from build123d import *

# Parameters (mm, degrees)
F1_DEPTH    = 16
F2_T        = 3
F2_T3_DEPTH = 22
F3_R        = 7.99999
F4_R        = 3.1035458613
F4_R_2      = 3.5498541614
F5_DEPTH    = 20


# Not quite as in the source:
# - a fillet or chamfer is up to 0.001 mm smaller than in the source, because OpenCascade refuses the exact size
# - a shell that OpenCascade refuses in one call is made with other operations: the cavity is built on its own and cut out


with BuildPart() as f1:
    # F0 (on Front) → F1 (new body)
    with BuildSketch(Plane.XZ):
        Polygon((-64.2090581298, 10), (-64.2090581298, 0), (31.7909418702, 0), (29.6909418702, 3), (24.7909418702, 10), (0.7909418702, 10), (-7.2090581298, 14), (-42.2090581298, 14), (-50.2090581298, 10), align=None)
        Polygon((31.7909418702, 0), (-64.2090581298, 0), (-64.2090581298, -10), (-50.2090581298, -10), (-42.2090581298, -14), (-7.2090581298, -14), (0.7909418702, -10), (24.7909418702, -10), (29.6909418702, -3), align=None)
        Polygon((29.6909418702, 3), (31.7909418702, 0), (29.6909418702, -3), (109.6909418702, -3), (109.6909418702, 3), align=None)
    extrude(amount=F1_DEPTH)

    # F2: shell of thickness 3, made by hand


with BuildPart() as f2_core1:
    # F2_t2: copy of F1
    add(f1.part)

    # the walls: a layer under each face that stays
    f2_faces = [f2_core1.faces().sort_by_distance(p)[0] for p in [
        (-24.7090581298, -8, 14),
        (-46.2090581298, -8, 12),
        (-57.2090581298, -8, 10),
        (-57.2090581298, -8, -10),
        (-46.2090581298, -8, -12),
        (-24.7090581298, -8, -14),
        (-3.2090581298, -8, -12),
        (12.7909418702, -8, -10),
        (27.2409418702, -8, -6.5),
        (69.6909418702, -8, -3),
        (109.6909418702, -8, 0),
        (69.6909418702, -8, 3),
        (27.2409418702, -8, 6.5),
        (12.7909418702, -8, 10),
        (-3.2090581298, -8, 12),
    ]]
    thicken(f2_faces, amount=-F2_T, mode=Mode.SUBTRACT)

    # F2_s4 → F2_t3 (cut)
    with BuildSketch(Plane.XZ.offset(-3)):
        Polygon((-50.2224745377, 10.0568328157), (-48.8674173433, 7.316718427), (-49.5008541973, 7), (-50.2090581298, 7), align=None)
        Polygon((-50.2224745377, -10.0568328157), (-50.2090581298, -7), (-49.5008541973, -7), (-48.8674173433, -7.316718427), align=None)
        Polygon((0.8043582781, -10.0568328157), (-0.5506989163, -7.316718427), (0.0827379377, -7), (0.7909418702, -7), align=None)
        Polygon((29.7155188278, -3.0472038703), (27.2332461087, -1.2796129669), (28.1289751855, 0), (29.6909418702, 0), align=None)
        Polygon((29.7155188278, 3.0472038703), (29.6909418702, 0), (28.1289751855, 0), (27.2332461087, 1.2796129669), align=None)
        Polygon((0.8043582781, 10.0568328157), (0.7909418702, 7), (0.0827379377, 7), (-0.5506989163, 7.316718427), align=None)
    extrude(amount=F2_T3_DEPTH, mode=Mode.SUBTRACT)


with BuildPart() as f1_1:
    add(f1.part)

    # what is left inside the walls is the cavity
    f2_cavity = [f2_core1.part.solids().sort_by_distance(p)[0] for p in [
        (-18.040041, -15.97, -3.666667),
    ]]
    add(f2_cavity, mode=Mode.SUBTRACT)

    # F3 (radius 8 in the source; OpenCascade refuses exactly that, so slightly less here)
    f3_edges = [f1_1.edges().sort_by_distance(p)[0] for p in [
        (-64.209058, -16, -8.5),
        (-64.209058, -16, 8.5),
        (-64.209058, 0, -8.5),
        (-64.209058, 0, 8.5),
        (109.690942, -16, 0),
        (109.690942, 0, 0),
    ]]
    fillet(f3_edges, radius=F3_R)

    # F4 (on face) → F5 (cut)
    with BuildSketch(Plane.XY.offset(10)):
        with Locations((-56.2090581298, -8)):
            Circle(F4_R)
        with Locations((6.7909418702, -7.7808454374)):
            Circle(F4_R_2)
    extrude(amount=-F5_DEPTH, mode=Mode.SUBTRACT)


solid = f1_1.part
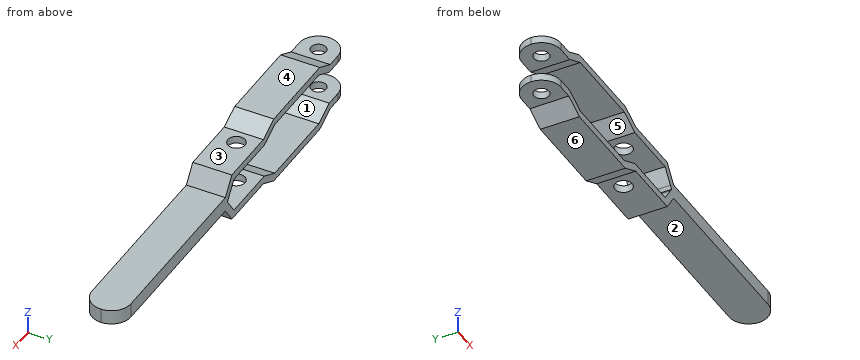
Check sheet for the modelled part. Datum: model origin and axes. Units: mm. Face numbers are marked on the shaded views. A direction names the side the tool comes from. Round coordinates to 2 decimals unless told otherwise and drop trailing zeros. Write each loop counter-clockwise with the first axis right and the second up, starting at its lowest first coordinate (ties: lowest second). Pieces come first, ordered by that corner, then holes. Notation, with made-up numbers: (4.5, 27.25) - (37.5, 27.25) arc R15 cw to (37.5, 38.25) - close; hole circle Ø4 at (0.25, 16.5). An arc over 180 degrees is marked (long way). Return JSON: item names as keys, results as strings.
Q1. Cross-section at C-C (z = 5.25). Record the boundary of the cut face in (x, y), then the cut area to 3 significant figures.
Returned:
{"outline": "(24.45, -16) - (28.12, -16) - (28.12, 0) - (24.45, 0) - close", "area": "58.6 mm²"}
Q2. Depth check by flat-ended pin: P1, Ø5, axis at y = -10.5, z = -3.5, coming from the -X side; P2, Ø1, axis at x = 91.5, y = -3.5, coming from the -Z side; P3, Ø8, axis at x = -56.21, y = -8, coming from the +Z side. Enter the tip coordinate at first touch or a pass-through.
Returned:
{"P1": "stops at x = 23.93", "P2": "stops at z = -3", "P3": "stops at z = 10"}
Q3. Cross-section at A-A (x = 48). Record the boundary of the cut face in (y, z).
Returned:
{"outline": "(-16, -3) - (0, -3) - (0, 3) - (-16, 3) - close"}
Q4. Scan lines: L1, parallel to Z at x = -33, y = -4.5; L2, parallel to Z at x = 22.5, y = -5.25; L3, parallel to Z at x = 57, y = -13.75. Record each from-to range of solid material in increasing order. Write a range as from..to.
Returned:
{"L1": "z = -14..-11, 11..14", "L2": "z = -10..-7, 7..10", "L3": "z = -3..3"}
Q5. Access from +Z, -Z, +X, -X, +Y, -Y to the whole of each face (thin tool, end or side, straight path). Record for the marked faces 1, 2 and 3.
Returned:
{"face 1": "+Y, -Y", "face 2": "-Z, +X, +Y, -Y", "face 3": "+Z, +X, +Y, -Y"}
Q6. Draft check along Z on the marked faces 4, 5 and 6. Enter one of: released by +Z, released by -Z, zero draft, split by the parting line, or undercut.
Returned:
{"face 4": "released by +Z", "face 5": "undercut", "face 6": "released by -Z"}
